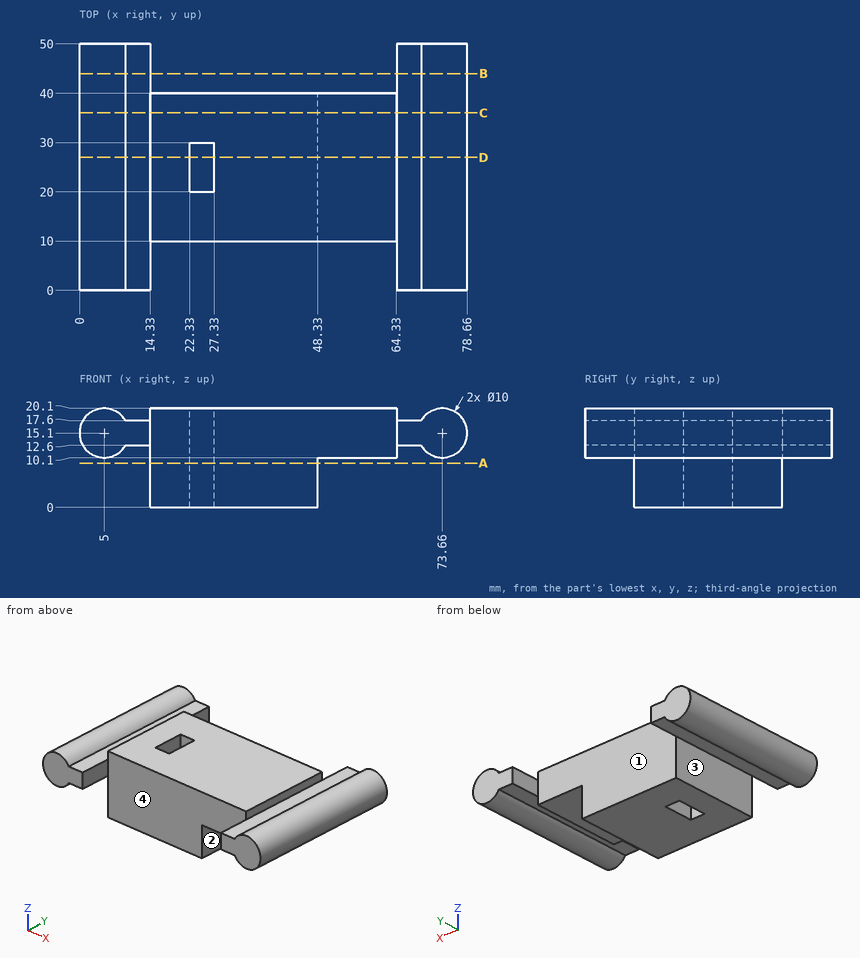
Geometry check sheet. Reference: drawing and pictorial views, mm from the part's lowest x, y, z. A direction names the side the tool comes from. Round coordinates to 2 decimals unless told otherwise and drop trailing zeros. Loops run counter-clockwise (first coordinate to the right, second up) from the corner with the lowest first, then second, coordinate; pieces in that order, holes last. Notation, with made-up numbers: (11, 71) - (42, 71) arc R35 cw to (42, 109) - close; hole circle Ø10 at (31, 11.25). An arc over 180 degrees is marked (long way). Use a Markdown table: item, result.
Q1. Go/stop test with flat-tipped pins: P1, Ø2, axis at x = 23.5, y = 24.5, coming from the -Z side; P2, Ø11, axis at y = 25.5, z = 7.5, coming from the +X side; P3, Ø1.2, axis at y = 29.5, z = 11.5, coming from the +X side; P4, Ø8, axis at y = 26.5, z = 6.5, coming from the -X side. Record where each tip stops, or that it passes through.
Solutions:
| item | result |
|---|---|
| P1 | passes through |
| P2 | stops at x = 78.2 |
| P3 | stops at x = 77.66 |
| P4 | stops at x = 3.04 |
Q2. Cross-section at B-B on y = 44. Record the cut outline in (x, z), plus the area to 3 significant figures.
Solutions:
| item | result |
|---|---|
| outline | (9.33, 12.6) - (14.33, 12.6) - (14.33, 17.6) - (9.33, 17.6) arc R5 ccw (long way) to start; (64.33, 12.6) - (69.33, 12.6) arc R5 ccw (long way) to (69.33, 17.6) - (64.33, 17.6) - close |
| area | 203 mm2 |
Q3. Cross-section at D-D on y = 27. Record the cut outline in (x, z).
Solutions:
| item | result |
|---|---|
| outline | (9.33, 12.6) - (14.33, 12.6) - (14.33, 0) - (22.33, 0) - (22.33, 20.1) - (14.33, 20.1) - (14.33, 17.6) - (9.33, 17.6) arc R5 ccw (long way) to start; (27.33, 0) - (48.33, 0) - (48.33, 10.1) - (64.33, 10.1) - (64.33, 12.6) - (69.33, 12.6) arc R5 ccw (long way) to (69.33, 17.6) - (64.33, 17.6) - (64.33, 20.1) - (27.33, 20.1) - close |
Q4. Material ranges on line 1 (Y direction, x = 23, z = 16); line 2 (X direction, y = 24, z = 11); line 3 (X direction, y = 29.5, z = 18), recorded low to high.
Solutions:
| item | result |
|---|---|
| line 1 | y = 10 to 20, 30 to 40 |
| line 2 | x = 2.14 to 7.86, 14.33 to 22.33, 27.33 to 64.33, 70.8 to 76.52 |
| line 3 | x = 0.93 to 9.07, 14.33 to 22.33, 27.33 to 64.33, 69.59 to 77.73 |
Q5. Access from +Z, -Z, +X, -X, +Y, -Y to the whole of each face (thin tool, end or side, straight path). Record for the marked faces 1, 2, 3 and 4.
Solutions:
| item | result |
|---|---|
| face 1 | +Z, -Z, +Y |
| face 2 | -Z, +X, +Y, -Y |
| face 3 | -Z, +Y, -Y |
| face 4 | +Z, -Z, -Y |
Q6. Cross-section at C-C on y = 36. Record the cut outline in (x, z).
Solutions:
| item | result |
|---|---|
| outline | (9.33, 12.6) - (14.33, 12.6) - (14.33, 0) - (48.33, 0) - (48.33, 10.1) - (64.33, 10.1) - (64.33, 12.6) - (69.33, 12.6) arc R5 ccw (long way) to (69.33, 17.6) - (64.33, 17.6) - (64.33, 20.1) - (14.33, 20.1) - (14.33, 17.6) - (9.33, 17.6) arc R5 ccw (long way) to start |
Q7. Cross-section at A-A on z = 9. Record the cut outline in (x, y).
Solutions:
| item | result |
|---|---|
| outline | (14.33, 10) - (48.33, 10) - (48.33, 40) - (14.33, 40) - close; hole (22.33, 20) - (27.33, 20) - (27.33, 30) - (22.33, 30) - close |
